Verification items for the finished model (mm, model axes). Round coordinates to 2 decimals unless told otherwise and drop trailing zeros. Order: outer loops, then holes, each group sorted by start corner. A loop starts at its lowest first (then second) coordinate and runs counter-clockwise, first axis right, second up. Notation, with made-up numbers: (1, 51) -> (41, 51) arc R9 ccw to (41, 59) -> close; hole circle Ø10 at (21, -4.5). An arc over 180 degrees is marked (long way). Return JSON: item names as keys, results as strings. Group by question number.
1) Scan lines: L1, parallel to X at y = 0.25, z = 1.2; L2, parallel to Y at x = -150, z = 1.7; L3, parallel to X at y = -2.25, z = 0.4. Record each from-to range of solid material in increasing order.
2) Section check B-B on z = 0.6. Enter the section's corners in (x, y), plus the area to 3 significant figures.
3) Section check A-A on y = 0. Enter the section's corners in (x, z).
4) Depth check by flat-ended pin: pin 1 (5 mm diameter, centred on x = -106.5, y = -3, fed in from -Z); pin 2 (1 mm diameter, centred on y = -3.5, z = 2, fed in from -X). Enter the tip coordinate at first touch or a pass-through.
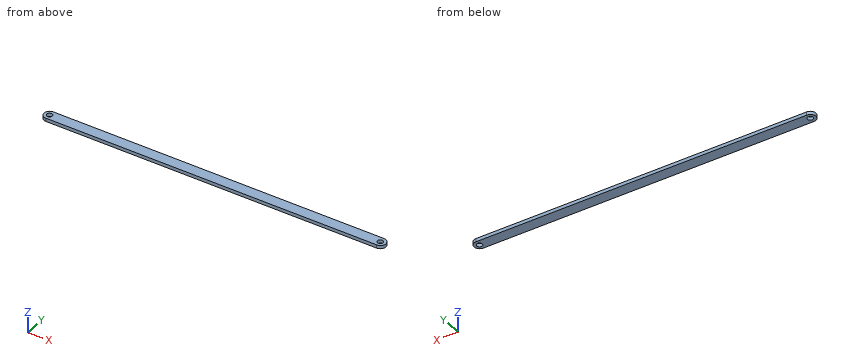
```python
from build123d import *

# Parameters (mm, degrees)
BOSS_EXTRUDE1_DEPTH = 3
CUT_EXTRUDE1_REACH  = 157.11
SKETCH2_R           = 2.5


with BuildPart() as part:
    # Sketch1 → Boss-Extrude1 (new body)
    with BuildSketch(Plane.XY):
        with BuildLine():
            Line((-150, 5), (150, 5))
            ThreePointArc((150, 5), (155, 0), (150, -5))
            Line((150, -5), (-150, -5))
            ThreePointArc((-150, -5), (-155, 0), (-150, 5))
        make_face()
    extrude(amount=BOSS_EXTRUDE1_DEPTH)

    # Sketch2 → Cut-Extrude1 (cut, up to next)
    with BuildSketch(Plane.XY.offset(3), mode=Mode.PRIVATE) as cut_extrude1_sk1:
        with Locations((-150, 0)):
            Circle(SKETCH2_R)
    cut_extrude1_tool1 = extrude(cut_extrude1_sk1.sketch, amount=-CUT_EXTRUDE1_REACH, mode=Mode.PRIVATE) & part.part
    cut_extrude1 = cut_extrude1_tool1.solids().sort_by_distance((-150, 0, 3))[0]
    add(cut_extrude1, mode=Mode.SUBTRACT)

    # Mirror1: Cut-Extrude1 across plane
    add(cut_extrude1.mirror(Plane(origin=(0, 0, 0), x_dir=(0, 0, 1), z_dir=(1, 0, 0))), mode=Mode.SUBTRACT)


solid = part.part
```
Check result:
{
 "1": {"L1": "-154.99 to -152.49, -147.51 to 147.51, 152.49 to 154.99", "L2": "-5 to -2.5, 2.5 to 5", "L3": "-154.47 to -151.09, -148.91 to 148.91, 151.09 to 154.47"},
 "2": {"outline": "(-150, -5) -> (150, -5) arc R5 ccw to (150, 5) -> (-150, 5) arc R5 ccw to start; hole circle Ø5 at (-150, 0); hole circle Ø5 at (150, 0)", "area": "3,040 mm^2"},
 "3": {"outline": "(-155, 0) -> (-152.5, 0) -> (-152.5, 3) -> (-155, 3) -> close; (-147.5, 0) -> (147.5, 0) -> (147.5, 3) -> (-147.5, 3) -> close; (152.5, 0) -> (155, 0) -> (155, 3) -> (152.5, 3) -> close"},
 "4": {"pin 1": "z = 0", "pin 2": "x = -154"}
}
